Build history of the part. All positions in model axes, mm. Round coordinates to 2 decimals unless told otherwise and drop trailing zeros. Write each loop counter-clockwise with the first axis right and the second up, starting at its lowest first coordinate (ties: lowest second). Pieces come first, ordered by that corner, then holes. Notation, with made-up numbers: (54.25, -23.5) - (104.25, -23.5) arc R24 cw to (104.25, 4.5) - close; hole circle Ø10 at (68, 84.25). An arc over 180 degrees is marked (long way). One line per question, with ' | ' between items.
from build123d import *

# Parameters (mm, degrees)
SKETCH_R               = 11
SKETCH_R_2             = 4
SKETCH_R_3             = 8
PAD_DEPTH              = 10.5
SKETCH001_R            = 22
SKETCH001_R_2          = 11
PAD001_DEPTH           = 27.5
SKETCH002_R            = 10
SKETCH002_R_2          = 4
SKETCH002_R_3          = 16
SKETCH002_R_4          = 8
PAD002_DEPTH           = 5
LINEARPATTERN_COUNT    = 2
LINEARPATTERN_PITCH    = 27.5
LINEARPATTERN001_COUNT = 2
LINEARPATTERN001_PITCH = 43


with BuildPart() as part:
    # Sketch → Pad (new body)
    with BuildSketch(Plane.XY):
        with BuildLine():
            ThreePointArc((-21.9234781804, 1.8333315232), (-9.5101896489, -19.8382532709), (15.1592048803, -15.9436039651))
            ThreePointArc((67.303030561, -8.8282771869), (40.0825387761, -3.968716444), (15.1592048803, -15.9436039651))
            ThreePointArc((67.303030561, -8.8282771869), (80.5823809431, -5.1325176421), (77.5552259696, 8.3150143973))
            ThreePointArc((77.5552259696, 8.3150143973), (54.1410477348, 19.8599663381), (28.5366090857, 24.9513688157))
            ThreePointArc((19.2247688114, 34.0968329356), (22.1829562344, 27.7954826606), (28.5366090857, 24.9513688157))
            Line((15.9443712103, 73.3330516519), (19.2247688114, 34.0968329356))
            ThreePointArc((15.9443712103, 73.3330516519), (0.000141406, 87.9999999994), (-15.9443476452, 73.3333334805))
            Line((-15.9443476452, 73.3333334805), (-21.9234781804, 1.8333315232))
        make_face()
        Circle(SKETCH_R, mode=Mode.SUBTRACT)
        with Locations((72, 0)):
            Circle(SKETCH_R_2, mode=Mode.SUBTRACT)
        with Locations((0, 72)):
            Circle(SKETCH_R_3, mode=Mode.SUBTRACT)
    pad = extrude(amount=PAD_DEPTH)

    # Sketch001 (on Face13 of Pad) → Pad001 (join)
    with BuildSketch(Plane.XY.offset(10.5)):
        Circle(SKETCH001_R)
        Circle(SKETCH001_R_2, mode=Mode.SUBTRACT)
    extrude(amount=PAD001_DEPTH)

    # Sketch002 (on Face4 of Pad001) → Pad002 (join)
    with BuildSketch(Plane(origin=(0, 0, 0), x_dir=(1, 0, 0), z_dir=(0, 0, -1))):
        with Locations((72, 0)):
            Circle(SKETCH002_R)
        with Locations((72, 0)):
            Circle(SKETCH002_R_2, mode=Mode.SUBTRACT)
        with Locations((0, -72)):
            Circle(SKETCH002_R_3)
        with Locations((0, -72)):
            Circle(SKETCH002_R_4, mode=Mode.SUBTRACT)
    pad002 = extrude(amount=PAD002_DEPTH)

    # LinearPattern: Pad ×2
    with Locations(*[(0, 0, i * LINEARPATTERN_PITCH) for i in range(1, LINEARPATTERN_COUNT)]):
        add(pad)

    # LinearPattern001: Pad002 ×2
    with Locations(*[(0, 0, i * LINEARPATTERN001_PITCH) for i in range(1, LINEARPATTERN001_COUNT)]):
        add(pad002)


solid = part.part
Q1. Pull direction Y, two halves, no side cores. Call faces 1 (the cylindrical face through (-1.041, 79.932, 2.641)), 2 (the cylindrical face through (-4.769, -21.477, 18.734)), 3 (the flat face through (-18.892, 38.084, 32.676)): +Y half, -Y half, draft (parallel to the pull), parting line (faces both ways), or undercut.
Found:
face 1: undercut | face 2: parting line | face 3: +Y half
Q2. Saw through at C-C, the plane z = 17. List the corners of the cut face in (x, y), then the cut area to 3 significant figures.
Found:
outline: circle Ø44 at (0, 0); hole circle Ø22 at (0, 0) | area: 1,140 mm^2
Q3. Saw through at D-D, the plane x = 46.5. List the corners of the cut face in (y, z), then the cut area to 3 significant figures.
Found:
outline: (-3.56, 0) - (22.12, 0) - (22.12, 10.5) - (-3.56, 10.5) - close; (-3.56, 27.5) - (22.12, 27.5) - (22.12, 38) - (-3.56, 38) - close | area: 539 mm^2
Q4. Saw through at A-A, the plane x = 72. List the corners of the cut face in (y, z), then the cut area to 3 significant figures.
Found:
outline: (-10, -5) - (-4, -5) - (-4, 10.5) - (-10, 10.5) - close; (-10, 27.5) - (-4, 27.5) - (-4, 43) - (-10, 43) - close; (4, -5) - (10, -5) - (10, 0) - (11.77, 0) - (11.77, 10.5) - (4, 10.5) - close; (4, 27.5) - (11.77, 27.5) - (11.77, 38) - (10, 38) - (10, 43) - (4, 43) - close | area: 409 mm^2
Q5. Saw through at B-B, the plane y = 0. List the corners of the cut face in (x, z).
Found:
outline: (-22, 0) - (-11, 0) - (-11, 38) - (-22, 38) - close; (11, 0) - (62, 0) - (62, -5) - (68, -5) - (68, 10.5) - (22, 10.5) - (22, 27.5) - (68, 27.5) - (68, 43) - (62, 43) - (62, 38) - (11, 38) - close; (76, -5) - (82, -5) - (82, 10.5) - (76, 10.5) - close; (76, 27.5) - (82, 27.5) - (82, 43) - (76, 43) - close
Q6. Drill centre lines: L1, parallel to Y at x = 0, z = 34.5; L2, parallel to Z at x = 27.5, y = 10.5; L3, parallel to Y at x = -6.5, z = 22. Where is each one in solid material? Low to high. Write a range as from..to.
Found:
L1: -22..-11, 11..64, 80..88 | L2: 0..10.5, 27.5..38 | L3: -21.02..-8.87, 8.87..21.02
Q7. Drop flat-ended pins along their axis: pin 1 (10 mm diameter, centred on y = 40, z = 31, fed in from -X); pin 2 (12 mm diameter, centred on y = -1, z = 9.5, fed in from +X); pin 3 (2 mm diameter, centred on y = 5.5, z = 3, fed in from -X); pin 4 (17.5 mm diameter, centred on x = 0, y = 0, fed in from -Z). Give the stop position or say it passes through.
Found:
pin 1: x = -19.15 | pin 2: x = 82 | pin 3: x = -21.7 | pin 4: through
